Could you check a few things on this model? Use its own coordinates, in mm. Give positions to 0.01 mm unless a question says otherwise; leave off trailing zeros. Loops run counter-clockwise (first coordinate to the right, second up) from the corner with the lowest first, then second, coordinate; pieces in that order, holes last. Notation, with made-up numbers: M 62.5,-32.75 L 99.5,-32.75 A19 ccw 99.5,-8.75 Z; hole C 9.25,9.5 d9. An arc over 180 degrees is marked long. Answer in a Markdown table with one row per item. Add a question column.
1. If we section it at A-A on y = 141: List the corners of the cut face in (x, z) for me, then the cut area to 3 significant figures.
2. I'm going to push flat-ended pins straight in: pin 1 Ø3 at (x, y) = (27.5, 74) entering from +Z; pin 2 Ø8 at (y, z) = (64, -14.5) entering from -X; pin 3 Ø12 at (x, y) = (21.5, 319) entering from +Z. Where does each tip first touch, or does it pass through?
3. If we section it at B-B on z = -70: List the corners of the cut face in (x, y) for me.
4. I need wall thicknesses on line 1 along X through (y, z) = (154.5, -22); line 2 along Z through (x, y) = (35, 189); line 3 along Z through (x, y) = (11.5, 431). Which ranges of each line are inside material? Lowest first, please. Write a range as from..to.
5. Thinking about a two-plate mould opening in Y: for faces 1 (the flat face through (63, -4.5, -66)), 2 (the flat face through (26, 504, -87)), 3 (the cylindrical face through (37.561, 489.308, -82.863)), which applies, released by +Y, released by -Y, zero draft, split by the parting line, or undercut?
```python
from build123d import *

# Parameters (mm, degrees)
BOSS_EXTRUDE1_DEPTH     = 508.5
CUT_EXTRUDE4_REACH      = 518.756
CUT_EXTRUDE4_END_RADIUS = 90
SKETCH6_R               = 5.565
CUT_EXTRUDE2_REACH      = 520.673
CUT_EXTRUDE2_END_RADIUS = 90
SKETCH3_R               = 5.565
CUT_EXTRUDE3_REACH      = 520.673
CUT_EXTRUDE3_END_RADIUS = 90
SKETCH5_R               = 5.565
LPATTERN2_COUNT         = 2
LPATTERN2_PITCH         = 488.5
CUT_EXTRUDE5_DEPTH      = 20
BODY_MOVE_COPY1_ANGLE   = 180


with BuildPart() as part:
    # Sketch1 → Boss-Extrude1 (new body)
    with BuildSketch(Plane(origin=(0, 0, 0), x_dir=(1, 0, 0), z_dir=(0, 1, 0))):
        with BuildLine():
            Line((0, 92), (0, 90))
            ThreePointArc((0, 90), (63.639610307, 63.639610307), (90, 0))
            Line((90, 0), (92, 0))
            ThreePointArc((92, 0), (65.053823869, 65.053823869), (0, 92))
        make_face()
    extrude(amount=BOSS_EXTRUDE1_DEPTH)

    # Cut-Extrude4: up to this cylinder (the profile starts outside it)
    cut_extrude4_end = Plane(origin=(0, 10, 0), z_dir=(0, -1, 0)) * Cylinder(CUT_EXTRUDE4_END_RADIUS, 1218.512, mode=Mode.PRIVATE)
    # Sketch6 → Cut-Extrude4 (cut, up to the surface)
    with BuildSketch(Plane(origin=(65.053823869, 0, -65.053823869), x_dir=(-0.7071067811865486, 0, -0.7071067811865465), z_dir=(0.7071067811865465, 0, -0.7071067811865486)), mode=Mode.PRIVATE) as cut_extrude4_sk1:
        with Locations((0, 10)):
            Circle(SKETCH6_R)
    cut_extrude4_tool1 = extrude(cut_extrude4_sk1.sketch, amount=-CUT_EXTRUDE4_REACH, mode=Mode.PRIVATE) - cut_extrude4_end
    add(cut_extrude4_tool1.solids().sort_by_distance((65.053824, 10, -65.053824))[0], mode=Mode.SUBTRACT)

    # Cut-Extrude2: up to this cylinder (the profile starts outside it)
    cut_extrude2_end = Plane(origin=(0, 10, 0), z_dir=(0, -1, 0)) * Cylinder(CUT_EXTRUDE2_END_RADIUS, 1222.346, mode=Mode.PRIVATE)
    # Sketch3 → Cut-Extrude2 (cut, up to the surface)
    with BuildSketch(Plane(origin=(84.996916991, 0, -35.206875778), x_dir=(-0.38268343236509045, 0, -0.9238795325112865), z_dir=(0.9238795325112865, 0, -0.38268343236509045)), mode=Mode.PRIVATE) as cut_extrude2_sk1:
        with Locations((0, 10)):
            Circle(SKETCH3_R)
    cut_extrude2_tool1 = extrude(cut_extrude2_sk1.sketch, amount=-CUT_EXTRUDE2_REACH, mode=Mode.PRIVATE) - cut_extrude2_end
    cut_extrude2 = cut_extrude2_tool1.solids().sort_by_distance((84.996917, 10, -35.206876))[0]
    add(cut_extrude2, mode=Mode.SUBTRACT)

    # Cut-Extrude3: up to this cylinder (the profile starts outside it)
    cut_extrude3_end = Plane(origin=(0, 10, 0), z_dir=(0, -1, 0)) * Cylinder(CUT_EXTRUDE3_END_RADIUS, 1222.346, mode=Mode.PRIVATE)
    # Sketch5 → Cut-Extrude3 (cut, up to the surface)
    with BuildSketch(Plane(origin=(35.206875778, 0, -84.996916991), x_dir=(-0.9238795325112878, 0, -0.3826834323650876), z_dir=(0.3826834323650876, 0, -0.9238795325112878)), mode=Mode.PRIVATE) as cut_extrude3_sk1:
        with Locations((0, 10)):
            Circle(SKETCH5_R)
    cut_extrude3_tool1 = extrude(cut_extrude3_sk1.sketch, amount=-CUT_EXTRUDE3_REACH, mode=Mode.PRIVATE) - cut_extrude3_end
    cut_extrude3 = cut_extrude3_tool1.solids().sort_by_distance((35.206876, 10, -84.996917))[0]
    add(cut_extrude3, mode=Mode.SUBTRACT)

    # LPattern2: Cut-Extrude2, Cut-Extrude3 ×2
    with Locations(*[(0, i * LPATTERN2_PITCH, 0) for i in range(1, LPATTERN2_COUNT)]):
        add(cut_extrude2, mode=Mode.SUBTRACT)
        add(cut_extrude3, mode=Mode.SUBTRACT)

    # Sketch7 → Cut-Extrude5 (cut)
    with BuildSketch(Plane.XZ):
        with BuildLine():
            Line((76.447375943, -51.183969281), (74.784435976, -50.072828318))
            ThreePointArc((74.784435976, -50.072828318), (63.639610307, -63.639610307), (50.072828318, -74.784435976))
            Line((50.072828318, -74.784435976), (51.183969281, -76.447375943))
            ThreePointArc((51.183969281, -76.447375943), (65.053823869, -65.053823869), (76.447375943, -51.183969281))
        make_face()
    extrude(amount=-CUT_EXTRUDE5_DEPTH, mode=Mode.SUBTRACT)


with BuildPart() as part_1:
    # Body-Move/Copy1: moved
    add(part.part.moved(Location((0, 0, 0))).rotate(Axis((0, 252, 0), (0.7071067811865488, -4.937700262164522e-15, -0.7071067811865462)), BODY_MOVE_COPY1_ANGLE))


solid = part_1.part
```
Results:
| question | item | result |
|---|---|---|
| 1 | outline | M 0,-92 A92 ccw 92,0 L 90,0 A90 cw 0,-90 Z |
| 1 | area | 286 mm2 |
| 2 | pin 1 | z = -85.2 |
| 2 | pin 2 | x = 88.08 |
| 2 | pin 3 | z = -85.7 |
| 3 | outline | M 56.57,-4.5 L 59.7,-4.5 L 59.7,484 L 56.57,484 Z |
| 4 | line 1 | 87.27..89.33 |
| 4 | line 2 | -85.08..-82.92 |
| 4 | line 3 | -91.28..-89.26 |
| 5 | face 1 | released by -Y |
| 5 | face 2 | released by +Y |
| 5 | face 3 | undercut |
